Design review of the part shown in the three views and the two pictorial views. Dimensions are in mm from the part's minimum x, y and z. Give positions to 0.01 mm unless a question says otherwise; leave off trailing zeros. Order: outer loops, then holes, each group sorted by start corner. A loop starts at its lowest first (then second) coordinate and runs counter-clockwise, first axis right, second up. Notation, with made-up numbers: (0.25, 14.25) -> (14.25, 14.25) arc R8 ccw to (14.25, 23.25) -> close; hole circle Ø10 at (-18.5, 70). An arc over 180 degrees is marked (long way). Use one line per item in the form item = value.
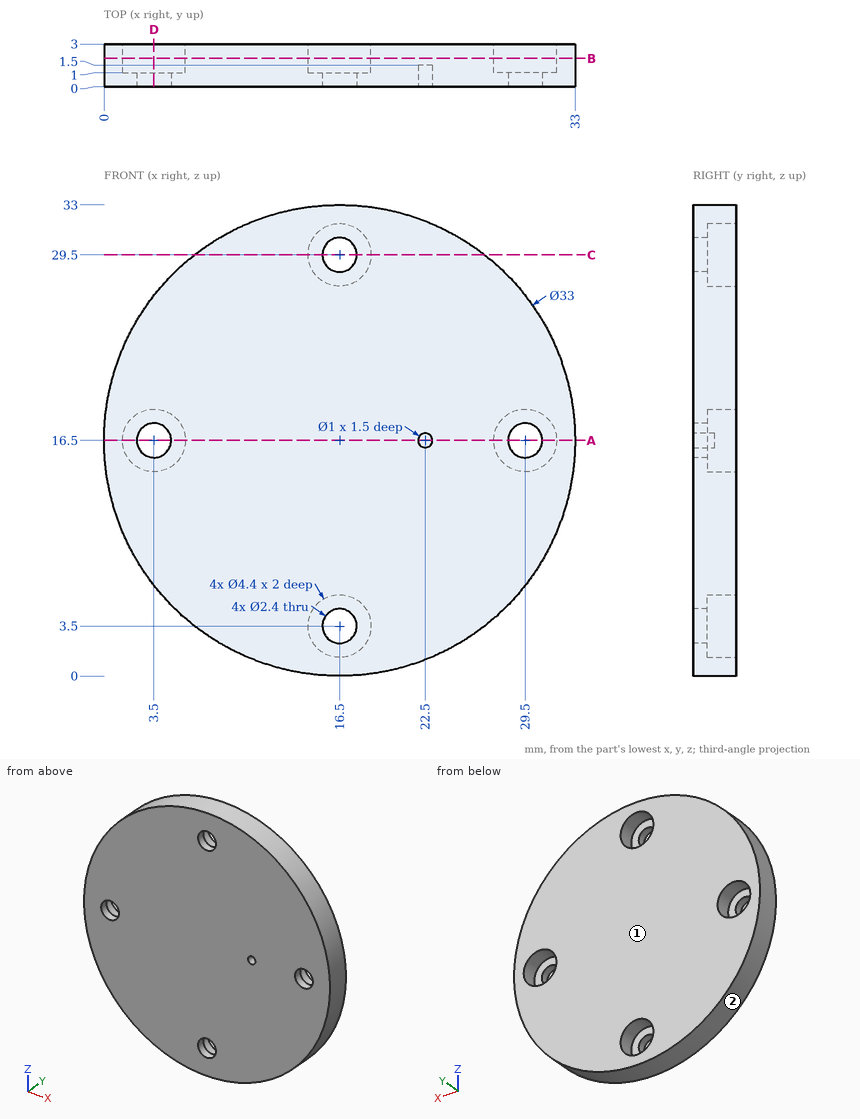
1. Add section B-B on y = 2. Give the boundary of the cut face in (x, z).
Values:
outline = circle Ø33 at (16.5, 16.5); hole circle Ø4.4 at (3.5, 16.5); hole circle Ø4.4 at (16.5, 3.5); hole circle Ø4.4 at (16.5, 29.5); hole circle Ø4.4 at (29.5, 16.5)
2. Add section D-D on x = 3.5. Give the boundary of the cut face in (y, z).
Values:
outline = (0, 6.34) -> (3, 6.34) -> (3, 14.3) -> (1, 14.3) -> (1, 15.3) -> (0, 15.3) -> close; (0, 17.7) -> (1, 17.7) -> (1, 18.7) -> (3, 18.7) -> (3, 26.66) -> (0, 26.66) -> close
3. For pin 1 Ø3.5 at (x, z) = (29.5, 16.5) entering from +Y; pin 2 Ø1 at (y, z) = (1.5, 5.5) entering from -X; pin 3 Ø2 at (x, z) = (16.5, 3.5) entering from +Y, all flat-tipped, find the tip position at first contact; note any pin that passes through.
Values:
pin_1 = 1
pin_2 = 3.77
pin_3 = through
4. Add section A-A on z = 16.5. Give the boundary of the cut face in (x, y).
Values:
outline = (0, 0) -> (2.3, 0) -> (2.3, 1) -> (1.3, 1) -> (1.3, 3) -> (0, 3) -> close; (4.7, 0) -> (22, 0) -> (22, 1.5) -> (23, 1.5) -> (23, 0) -> (28.3, 0) -> (28.3, 1) -> (27.3, 1) -> (27.3, 3) -> (5.7, 3) -> (5.7, 1) -> (4.7, 1) -> close; (30.7, 0) -> (33, 0) -> (33, 3) -> (31.7, 3) -> (31.7, 1) -> (30.7, 1) -> close
5. Add section C-C on z = 29.5. Give the boundary of the cut face in (x, y), then the cut area to 3 significant figures.
Values:
outline = (6.34, 0) -> (15.3, 0) -> (15.3, 1) -> (14.3, 1) -> (14.3, 3) -> (6.34, 3) -> close; (17.7, 0) -> (26.66, 0) -> (26.66, 3) -> (18.7, 3) -> (18.7, 1) -> (17.7, 1) -> close
area = 49.8 mm^2
6. For L1, parallel to Z at x = 3, y = 1.5; L2, parallel to X at y = 1.8, z = 4.5; L3, parallel to X at y = 1.2, z = 5.5, list the stretches that pass through material, from the lowest coordinate up.
Values:
L1 = 7.01 to 14.36, 18.64 to 25.99
L2 = 5.18 to 14.54, 18.46 to 27.82
L3 = 4.2 to 15.58, 17.42 to 28.8
7. The part is to be moulded in two halves that separate along Z. For the marked faces 1 and 2, say which applies: +Z half, -Z half, draft (parallel to the pull), parting line (faces both ways), or undercut.
Values:
face_1 = draft
face_2 = parting line
